```python
from build123d import *

# Parameters (mm, degrees)
F3_DEPTH = 12.5


with BuildPart() as f1:
    # F0 (on Front) → F1 (revolve)
    with BuildSketch(Plane.XZ):
        Polygon((0, 0), (0, 27), (-42, 24), (-42, 0), align=None)
    revolve(axis=Axis((-21, 0, 0), (1, 0, 0)))

    # F2 (on Front) → F3 (join, symmetric)
    with BuildSketch(Plane.XZ):
        with BuildLine():
            ThreePointArc((-18.532742, 40.028698), (-28.904432, 31.158633), (-42, 35))
            Line((-42, 35), (-42, 0))
            Line((-42, 0), (-18.532742, 0))
            Line((-18.532742, 0), (-18.532742, 40.028698))
        make_face()
    extrude(amount=F3_DEPTH, both=True)


solid = f1.part
```
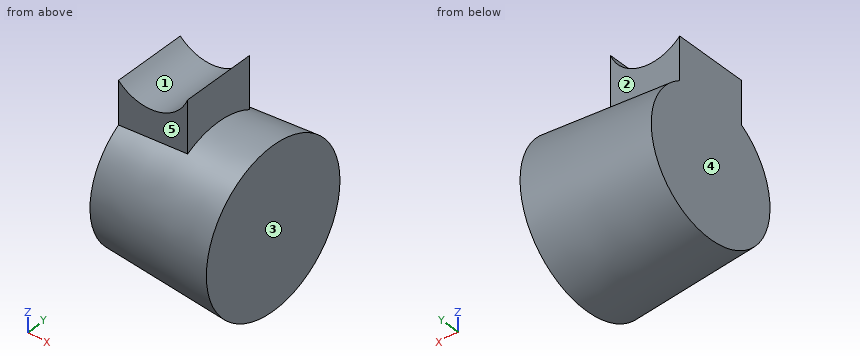
Here's how the part is built. I have some questions about the finished solid (model axes, mm). Face numbers are marked on the shaded views. A direction names the side the tool comes from. Give positions to 0.01 mm unless a question says otherwise; leave off trailing zeros. Write each loop counter-clockwise with the first axis right and the second up, starting at its lowest first coordinate (ties: lowest second). Pieces come first, ordered by that corner, then holes. Notation, with made-up numbers: (81, 69) -> (122, 69) arc R37 cw to (122, 105) -> close; hole circle Ø2 at (38.25, 67). An arc over 180 degrees is marked (long way). Write each question's results on one line, items separated by ' | '.
Item 1: Suppose I cut it at D-D on x = -25. Write out the boundary of the cut face in (y, z).
Output:
outline: (-12.5, 21.9) arc R25.21 ccw (long way) to (12.5, 21.9) -> (12.5, 32.62) -> (-12.5, 32.62) -> close
Item 2: Suppose I cut it at C-C on y = 0. Write out the boundary of the cut face in (x, z), plus the area to 3 significant figures.
Output:
outline: (-42, -24) -> (0, -27) -> (0, 27) -> (-18.53, 25.68) -> (-18.53, 40.03) arc R14.33 cw to (-42, 35) -> close | area: 2,330 mm^2
Item 3: Suppose I cut it at A-A on z = 34. Write out the boundary of the cut face in (x, y), plus the area to 3 significant figures.
Output:
outline: (-42, -12.5) -> (-40.88, -12.5) -> (-40.88, 12.5) -> (-42, 12.5) -> close; (-22.93, -12.5) -> (-18.53, -12.5) -> (-18.53, 12.5) -> (-22.93, 12.5) -> close | area: 138 mm^2
Item 4: If I drill on L1, parallel to Z at x = -35.5, y = 0; L2, parallel to Y at x = -9, z = 10.5; L3, parallel to Z at x = -3.5, y = -11, over which ranges is the centre line in solid material (lowest first)?
Output:
L1: z = -24.46 to 31.3 | L2: y = -24.18 to 24.18 | L3: z = -24.38 to 24.38
Item 5: We'd pull the mould along X, two halves only. Please class the marked faces 1, 2 and 3: pulls with the +X half, pulls with the -X half, needs draft (parallel to the pull), parting line crosses it, or undercut.
Output:
face 1: undercut | face 2: needs draft | face 3: pulls with the +X half
Item 6: On a 3-axis mill with a long thin cutter (end or side, diameter ignored), from which of +Z, -Z, +X, -X, +Y, -Y can I reach the whole of each face in a straight line? I mean the marked faces 4 and 5. Say none if no direction works.
Output:
face 4: +Z, -Z, -X, +Y, -Y | face 5: +Z, -X, -Y
Item 7: For pin 1 Ø1.5 at (x, y) = (-31, -9.5) entering from -Z; pin 2 Ø8 at (x, y) = (-10.5, 11.5) entering from -Z; pin 3 Ø10 at (x, z) = (-36, 24.5) entering from +Y, each with a flat end and sliding along its axis, tell me the tip position at first contact or that it passes through.
Output:
pin 1: stops at z = -23.2 | pin 2: stops at z = -25.19 | pin 3: stops at y = 14.74
Item 8: Suppose I cut it at B-B on z = 0. Write out the boundary of the cut face in (x, y).
Output:
outline: (-42, -24) -> (0, -27) -> (0, 27) -> (-42, 24) -> close
